Source: three-view drawing plus pictorial views. Frame: mm from the lowest corner of the part. Coordinates: 2 decimals unless noted, no trailing zeros. Loops run counter-clockwise (first coordinate to the right, second up) from the corner with the lowest first, then second, coordinate; pieces in that order, holes last. Notation, with made-up numbers: (40.5, -4.5) - (49.5, -4.5) arc R27 ccw to (49.5, 22.5) - close; hole circle Ø7 at (51.25, 22). An arc over 180 degrees is marked (long way). Return JSON: item names as keys, results as strings.
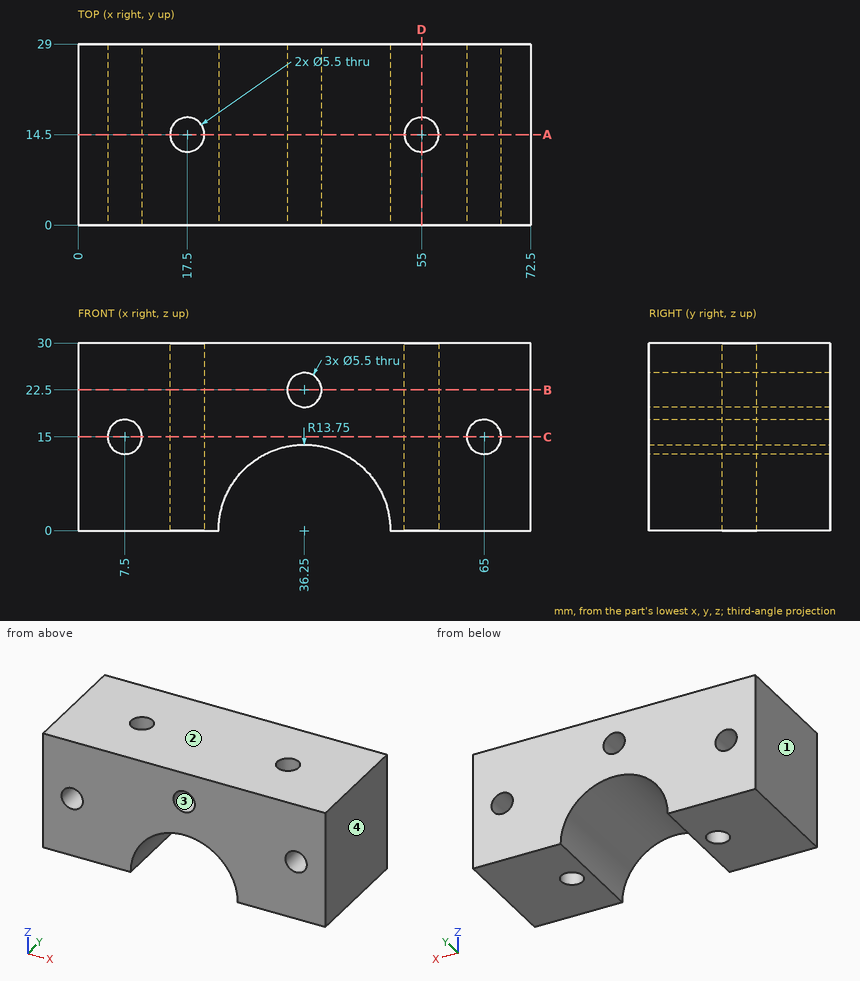
Item 1: Ray query, probe 1 along Y at (x, z) = (17.5, 18.5); probe 2 along X at (y, z) = (24.75, 17); probe 3 along X at (y, z) = (13.5, 18.75). Return the intervals inside material, ascending. Write a range as from..to.
Worked out:
{"probe 1": "0..11.75, 17.25..29", "probe 2": "0..5.61, 9.39..63.11, 66.89..72.5", "probe 3": "0..14.94, 20.06..52.44, 57.56..72.5"}
Item 2: Section query D-D, the plane x = 55. Return loops of the section in (y, z).
Worked out:
{"outline": "(0, 0) - (11.75, 0) - (11.75, 30) - (0, 30) - close; (17.25, 0) - (29, 0) - (29, 30) - (17.25, 30) - close"}
Item 3: First-contact query: pin 1 Ø5 at (x, z) = (7.5, 15) entering from -Y. Flat tip, straight axial feed; report the tip coordinate or a pass-through.
Worked out:
{"pin 1": "through"}
Item 4: Section query A-A, the plane y = 14.5. Return loops of the section in (x, z).
Worked out:
{"outline": "(0, 0) - (14.75, 0) - (14.75, 30) - (0, 30) - close; (20.25, 0) - (22.5, 0) arc R13.75 cw to (50, 0) - (52.25, 0) - (52.25, 30) - (20.25, 30) - close; (57.75, 0) - (72.5, 0) - (72.5, 30) - (57.75, 30) - close; hole circle Ø5.5 at (7.5, 15); hole circle Ø5.5 at (36.25, 22.5); hole circle Ø5.5 at (65, 15)"}
Item 5: Section query C-C, the plane z = 15. Return loops of the section in (x, y).
Worked out:
{"outline": "(0, 0) - (4.75, 0) - (4.75, 29) - (0, 29) - close; (10.25, 0) - (62.25, 0) - (62.25, 29) - (10.25, 29) - close; (67.75, 0) - (72.5, 0) - (72.5, 29) - (67.75, 29) - close; hole circle Ø5.5 at (17.5, 14.5); hole circle Ø5.5 at (55, 14.5)"}
Item 6: Mould query, pull axis X, two halves, no side actions, for the marked faces 1, 2, 3 and 4. Classes: +X half, -X half, draft (parallel to the pull), parting line (faces both ways), or undercut.
Worked out:
{"face 1": "-X half", "face 2": "draft", "face 3": "undercut", "face 4": "+X half"}
Item 7: Section query B-B, the plane z = 22.5. Return loops of the section in (x, y).
Worked out:
{"outline": "(0, 0) - (33.5, 0) - (33.5, 29) - (0, 29) - close; (39, 0) - (72.5, 0) - (72.5, 29) - (39, 29) - close; hole circle Ø5.5 at (17.5, 14.5); hole circle Ø5.5 at (55, 14.5)"}
